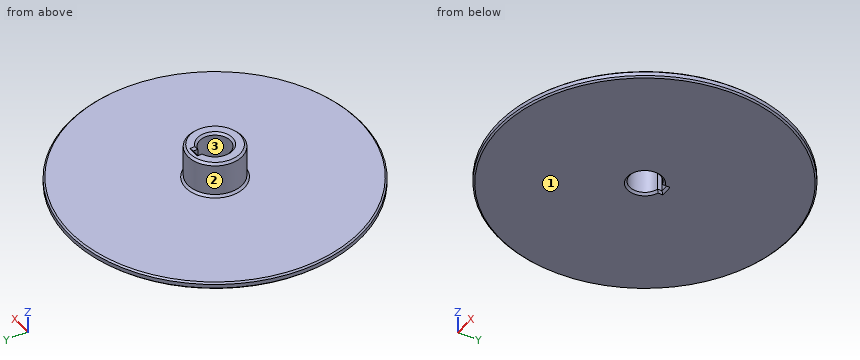
```python
from build123d import *

# Parameters (mm, degrees)
SKETCH1_R               = 121.331498574
BOSS_EXTRUDE1_DEPTH     = 5.7658
SKETCH2_R               = 22.479
BOSS_EXTRUDE2_DEPTH     = 29.174948
CUT_EXTRUDE1_DEPTH      = 176.110025307
CUT_EXTRUDE1_DEPTH_BACK = 176.110025307
SKETCH3_R               = 12.7
CUT_EXTRUDE2_DEPTH      = 176.110025307
CUT_EXTRUDE2_DEPTH_BACK = 176.110025307
SKETCH4_W               = 6.35
SKETCH4_H               = 6.35
CHAMFER1_SIZE           = 1.27
CHAMFER2_SIZE           = 1.778


with BuildPart() as part:
    # Sketch1 → Boss-Extrude1 (new body)
    with BuildSketch(Plane.XY):
        with Locations(Location((0, 0, 0), (0, 0, 180))):
            Circle(SKETCH1_R)
    extrude(amount=BOSS_EXTRUDE1_DEPTH)

    # Sketch2 → Boss-Extrude2 (add)
    with BuildSketch(Plane.XY.offset(5.7658)):
        with Locations(Location((0, 0, 0), (0, 0, 180))):
            Circle(SKETCH2_R)
    extrude(amount=BOSS_EXTRUDE2_DEPTH)

    # Sketch3 → Cut-Extrude1 (cut, two sides: drawn at the far end of the back side and taken through both)
    with BuildSketch(Plane.XY.offset(34.940748).offset(-CUT_EXTRUDE1_DEPTH_BACK)):
        Circle(SKETCH3_R)
    extrude(amount=CUT_EXTRUDE1_DEPTH + CUT_EXTRUDE1_DEPTH_BACK, mode=Mode.SUBTRACT)

    # Sketch4 → Cut-Extrude2 (cut, two sides: drawn at the far end of the back side and taken through both)
    with BuildSketch(Plane.XY.offset(34.940748).offset(-CUT_EXTRUDE2_DEPTH_BACK)):
        with Locations((0, 12.7)):
            Rectangle(SKETCH4_W, SKETCH4_H)
    extrude(amount=CUT_EXTRUDE2_DEPTH + CUT_EXTRUDE2_DEPTH_BACK, mode=Mode.SUBTRACT)

    # Chamfer1
    chamfer1_edges = [part.edges().sort_by_distance(p)[0] for p in [
        (121.331498574, 0, 0),
        (121.331498574, 0, 5.7658),
    ]]
    chamfer(chamfer1_edges, length=CHAMFER1_SIZE)

    # Chamfer2
    chamfer2_edges = [part.edges().sort_by_distance(p)[0] for p in [
        (0, -12.7, 34.940748),
        (0, -12.7, 0),
        (0, 15.875, 34.940748),
        (3.175, 14.085861062, 34.940748),
        (-3.175, 14.085861062, 34.940748),
        (3.175, 14.085861062, 0),
        (-3.175, 14.085861062, 0),
        (0, 15.875, 0),
        (22.479, 0, 5.7658),
        (22.479, 0, 34.940748),
    ]]
    chamfer(chamfer2_edges, length=CHAMFER2_SIZE)


solid = part.part
```
Source: CAD feature listing. Evaluate the final solid. Frame: model axes, mm. Face numbers are marked on the shaded views. Round coordinates to 2 decimals unless told otherwise and drop trailing zeros. Loops run counter-clockwise (first coordinate to the right, second up) from the corner with the lowest first, then second, coordinate; pieces in that order, holes last.
(1) Pull-direction query (Y, two-part tool) for the marked faces 1, 2 and 3; classes: +Y half, -Y half, draft (parallel to the pull), parting line (faces both ways), or undercut.
From the geometry:
face 1: draft
face 2: parting line
face 3: undercut
(2) Section query C-C (z = 20.5). Output: boundary loops of the cut face in (x, y) (3 decimals), and give its area (3 significant figures).
From the geometry:
outline: circle Ø44.958 at (0, 0); hole (-3.175, 12.297) arc R12.7 ccw (long way) to (3.175, 12.297) - (3.175, 15.875) - (-3.175, 15.875) - close
area: 1,060 mm2
(3) Section query A-A (y = 0). Output: boundary loops of the cut face in (x, z), and give its area (3 significant figures).
From the geometry:
outline: (-121.33, 1.27) - (-120.06, 0) - (-14.48, 0) - (-12.7, 1.78) - (-12.7, 33.16) - (-14.48, 34.94) - (-20.7, 34.94) - (-22.48, 33.16) - (-22.48, 7.54) - (-24.26, 5.77) - (-120.06, 5.77) - (-121.33, 4.5) - close; (12.7, 1.78) - (14.48, 0) - (120.06, 0) - (121.33, 1.27) - (121.33, 4.5) - (120.06, 5.77) - (24.26, 5.77) - (22.48, 7.54) - (22.48, 33.16) - (20.7, 34.94) - (14.48, 34.94) - (12.7, 33.16) - close
area: 1,810 mm2
(4) Contact query for flat-ended pins moving along their axis: pin 1 Ø12 at (y, z) = (-4.5, 26) entering from +X; pin 2 Ø1.1 at (y, z) = (14, 11.5) entering from -X; pin 3 Ø3 at (y, z) = (10.5, 7) entering from -X. Output: stop coordinate, or through.
From the geometry:
pin 1: stops at x = 22.48
pin 2: stops at x = -18.01
pin 3: stops at x = -119.87
(5) Section query B-B (x = 0). Output: boundary loops of the cut face in (y, z) (1 decimal), and give its area (3 significant figures).
From the geometry:
outline: (-121.3, 1.3) - (-120.1, 0) - (-14.5, 0) - (-12.7, 1.8) - (-12.7, 33.2) - (-14.5, 34.9) - (-20.7, 34.9) - (-22.5, 33.2) - (-22.5, 7.5) - (-24.3, 5.8) - (-120.1, 5.8) - (-121.3, 4.5) - close; (15.9, 1.8) - (17.7, 0) - (120.1, 0) - (121.3, 1.3) - (121.3, 4.5) - (120.1, 5.8) - (24.3, 5.8) - (22.5, 7.5) - (22.5, 33.2) - (20.7, 34.9) - (17.7, 34.9) - (15.9, 33.2) - close
area: 1,700 mm2
(6) Material intervals for probe 1 along Y at (x, z) = (1, 4) (3 decimals); probe 2 along Y at (x, z) = (0, 16) (3 decimals); probe 3 along Z at (x, y) = (10.5, 76), sorted ascending.
From the geometry:
probe 1: y = -121.327 to -12.661, 15.875 to 121.327
probe 2: y = -22.479 to -12.7, 15.875 to 22.479
probe 3: z = 0 to 5.77
